Could you check a few things on this model? Use its own coordinates, in mm. Face numbers are marked on the shaded views. A direction names the side the tool comes from. Coordinates: 2 decimals unless noted, no trailing zeros. Write each loop counter-clockwise with the first axis right and the second up, starting at its lowest first coordinate (ties: lowest second). Pieces come first, ordered by that corner, then holes. Notation, with made-up numbers: M 31.5,82 L 77.5,82 A19 cw 77.5,103 Z; hole C 85,-26 d2. An arc over 180 degrees is marked long. Write item = value, one per line.
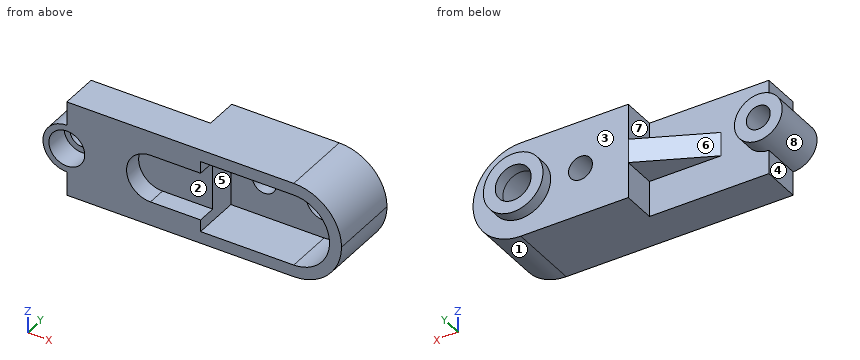
```python
from build123d import *

# Parameters (mm, degrees)
SKETCH1_W               = 115
SKETCH1_H               = 40
BOSS_EXTRUDE1_DEPTH     = 16
SKETCH2_R               = 10
SKETCH2_R_2             = 5
BOSS_EXTRUDE2_DEPTH     = 23
SKETCH3_R               = 7.5
CUT_EXTRUDE1_DEPTH      = 10
CUT_EXTRUDE2_DEPTH      = 36
CUT_EXTRUDE2_DEPTH_BACK = 24
SKETCH4_R               = 5
SKETCH5_W               = 65
SKETCH5_H               = 40
BOSS_EXTRUDE3_DEPTH     = 14
RIB2_REACH              = 78.526
SKETCH8_WALL_W          = 188.158169364
SKETCH8_WALL_H          = 10
FILLET3_R               = 20
SKETCH10_R              = 12.5
SKETCH10_R_2            = 7.5
BOSS_EXTRUDE4_DEPTH     = 5
SKETCH11_R              = 7.5
CUT_EXTRUDE3_DEPTH      = 77.526139325
SKETCH12_R              = 5
CUT_EXTRUDE4_DEPTH      = 77.526139325
CUT_EXTRUDE5_DEPTH      = 20
CUT_EXTRUDE6_DEPTH      = 8


with BuildPart() as part:
    # Sketch1 → Boss-Extrude1 (new body)
    with BuildSketch(Plane(origin=(0, 0, 0), x_dir=(1, 0, 0), z_dir=(0, 1, 0))):
        Rectangle(SKETCH1_W, SKETCH1_H)
    extrude(amount=BOSS_EXTRUDE1_DEPTH)

    # Sketch2 → Boss-Extrude2 (add)
    with BuildSketch(Plane(origin=(0, 0, 0), x_dir=(1, 0, 0), z_dir=(0, 1, 0))):
        with Locations(Location((-57.5, 0, 0), (0, 0, 270))):
            Circle(SKETCH2_R)
        with Locations(Location((-57.5, 0, 0), (0, 0, 270))):
            Circle(SKETCH2_R_2, mode=Mode.SUBTRACT)
    extrude(amount=BOSS_EXTRUDE2_DEPTH)

    # Sketch3 → Cut-Extrude1 (cut)
    with BuildSketch(Plane(origin=(0, 0, 0), x_dir=(1, 0, 0), z_dir=(0, 1, 0))):
        with Locations(Location((-57.5, 0, 0), (0, 0, 270))):
            Circle(SKETCH3_R)
    extrude(amount=CUT_EXTRUDE1_DEPTH, mode=Mode.SUBTRACT)

    # Sketch4 → Cut-Extrude2 (cut, two sides: drawn at the far end of the back side and taken through both)
    with BuildSketch(Plane(origin=(0, 0, 0), x_dir=(1, 0, 0), z_dir=(0, 1, 0)).offset(-CUT_EXTRUDE2_DEPTH_BACK)):
        with Locations(Location((-57.5, 0, 0), (0, 0, 270))):
            Circle(SKETCH4_R)
    extrude(amount=CUT_EXTRUDE2_DEPTH + CUT_EXTRUDE2_DEPTH_BACK, mode=Mode.SUBTRACT)

    # Sketch5 → Boss-Extrude3 (add)
    with BuildSketch(Plane(origin=(0, 16, 0), x_dir=(1, 0, 0), z_dir=(0, 1, 0))):
        with Locations((25, 0)):
            Rectangle(SKETCH5_W, SKETCH5_H)
    extrude(amount=BOSS_EXTRUDE3_DEPTH)

    # Sketch8 wall → Rib2 (add, up to next)
    with BuildSketch(Plane(origin=(-22.5, 23, 0), x_dir=(0.906183139995, 0.422885465331, 0), z_dir=(-0.422885465331, 0.906183139995, 0)), mode=Mode.PRIVATE) as rib2_sk1:
        Rectangle(SKETCH8_WALL_W, SKETCH8_WALL_H)
    rib2_tool1 = extrude(rib2_sk1.sketch, amount=-RIB2_REACH, mode=Mode.PRIVATE) - part.part
    add(rib2_tool1.solids().sort_by_distance((-22.5, 23, 0))[0])

    # Fillet3
    fillet3_edges = [part.edges().sort_by_distance(p)[0] for p in [
        (57.5, 15, -20),
        (57.5, 15, 20),
    ]]
    fillet(fillet3_edges, radius=FILLET3_R - 0.0001)  # a hair under: the kernel refuses the full size

    # Sketch10 → Boss-Extrude4 (add)
    with BuildSketch(Plane(origin=(0, 30, 0), x_dir=(1, 0, 0), z_dir=(0, 1, 0))):
        with Locations(Location((37.5, 0, 0), (0, 0, 90))):
            Circle(SKETCH10_R)
        with Locations(Location((37.5, 0, 0), (0, 0, 270))):
            Circle(SKETCH10_R_2, mode=Mode.SUBTRACT)
    extrude(amount=BOSS_EXTRUDE4_DEPTH)

    # Sketch11 → Cut-Extrude3 (cut, through all)
    with BuildSketch(Plane(origin=(0, 30, 0), x_dir=(1, 0, 0), z_dir=(0, 1, 0))):
        with Locations(Location((37.5, 0, 0), (0, 0, 270))):
            Circle(SKETCH11_R)
    extrude(amount=-CUT_EXTRUDE3_DEPTH, mode=Mode.SUBTRACT)

    # Sketch12 → Cut-Extrude4 (cut, through all)
    with BuildSketch(Plane(origin=(0, 30, 0), x_dir=(1, 0, 0), z_dir=(0, 1, 0))):
        with Locations(Location((12.5, 0, 0), (0, 0, 270))):
            Circle(SKETCH12_R)
    extrude(amount=-CUT_EXTRUDE4_DEPTH, mode=Mode.SUBTRACT)

    # Sketch13 → Cut-Extrude5 (cut)
    with BuildSketch(Plane(origin=(0, 0, 0), x_dir=(1, 0, 0), z_dir=(0, 1, 0))):
        with BuildLine():
            Line((37.5, -15), (-1.5, -15))
            Line((-1.5, -15), (-1.5, 15))
            Line((-1.5, 15), (37.5, 15))
            ThreePointArc((37.5, 15), (52.5, 0), (37.5, -15))
        make_face()
    extrude(amount=CUT_EXTRUDE5_DEPTH, mode=Mode.SUBTRACT)

    # Sketch14 → Cut-Extrude6 (cut)
    with BuildSketch(Plane(origin=(0, 0, 0), x_dir=(1, 0, 0), z_dir=(0, 1, 0))):
        with BuildLine():
            Line((-22.5, 10), (-1.5, 10))
            Line((-1.5, 10), (-1.5, -10))
            Line((-1.5, -10), (-22.5, -10))
            ThreePointArc((-22.5, -10), (-32.5, 0), (-22.5, 10))
        make_face()
    extrude(amount=CUT_EXTRUDE6_DEPTH, mode=Mode.SUBTRACT)


solid = part.part
```
Item 1: If I drill on line 1 along X through (y, z) = (3.25, 0); line 2 along Z through (x, y) = (12, 23); line 3 along X through (y, z) = (26, 0), over which ranges is the centre line in solid material (lowest first)?
Numbers:
line_1 = -67.5 to -65, -50 to -32.5, 52.5 to 57.5
line_2 = -20 to -4.97, 4.97 to 20
line_3 = -16.07 to 7.5, 17.5 to 30, 45 to 57.5
Item 2: Imagine slicing it at B-B (y = 26.5). State how many separate pieces and enclosed holes the cut face has, and give its area (3 significant figures).
Numbers:
separate_pieces = 1
enclosed_holes = 2
area = 2,250 mm²
Item 3: I'm going to push flat-ended pins straight in: P1, Ø15.5, axis at x = -16, y = 25.5, coming from the +Z side; P2, Ø17, axis at x = -57.5, z = 0, coming from the -Y side; P3, Ø3, axis at x = -51.5, z = 3.5, coming from the +Y side; P4, Ø7, axis at x = -17, y = 20, coming from the -Z side. Where does each tip first touch, or does it pass through?
Numbers:
P1 = 5
P2 = 0
P3 = 23
P4 = -5
Item 4: Imagine slicing it at A-A (x = 12.5). Write out the boundary of the cut face in (y, z).
Numbers:
outline = M 0,-20 L 30,-20 L 30,-5 L 20,-5 L 20,-15 L 0,-15 Z; M 0,15 L 20,15 L 20,5 L 30,5 L 30,20 L 0,20 Z
Item 5: If we mould it in two halves opening along X, with no side actions, what happens to the marked faces 1, 2 and 3? For each: pulls with the +X half, pulls with the -X half, needs draft (parallel to the pull), parting line crosses it, or undercut.
Numbers:
face_1 = pulls with the +X half
face_2 = undercut
face_3 = needs draft
Item 6: For the marked faces 4, 5, 6, 7 and 8, which set-ups out of +Z, -Z, +X, -X, +Y, -Y let a thin tool reach every point of the face, with its end or its side?
Numbers:
face_4 = -Z, -X, +Y, -Y
face_5 = -Y
face_6 = +Z, -Z, +Y
face_7 = +Z, +Y
face_8 = +Y
